```python
from build123d import *

# Parameters (mm, degrees)
SPLIT_2_DEPTH      = 10
SPLIT_2_DEPTH_BACK = 40.867646096
SPLSKE_W           = 5.7748
SPLSKE_H           = 1.850215418


with BuildPart() as part:
    # BodySke → Body (revolve)
    with BuildSketch(Plane.XY, mode=Mode.PRIVATE) as body_sk:
        with BuildLine():
            Line((0, 2.5), (38.74, 2.8874))
            ThreePointArc((38.74, 2.8874), (39.422958568, 1.514905806), (39.65797584, 0))
            Line((39.65797584, 0), (-0.669872981, 0))
            ThreePointArc((-0.669872981, 0), (-0.499502113, 1.294095226), (0, 2.5))
        make_face()
    revolve(body_sk.sketch.rotate(Axis((-0.669872981, 0, 0), (1, 0, 0)), 90), axis=Axis((-0.669872981, 0, 0), (1, 0, 0)))

    # SplSke → Split 2 (cut, two sides: drawn at the far end of the back side and taken through both)
    with BuildSketch(Plane(origin=(0, 0, 0), x_dir=(0, 0, -1), z_dir=(1, 0, 0)).offset(-SPLIT_2_DEPTH_BACK)):
        Rectangle(SPLSKE_W, SPLSKE_H)
    extrude(amount=SPLIT_2_DEPTH + SPLIT_2_DEPTH_BACK, mode=Mode.SUBTRACT)


solid = part.part
```
Verification items for the finished model (mm, model axes). Coordinates: 2 decimals unless noted, no trailing zeros. Loops run counter-clockwise (first coordinate to the right, second up) from the corner with the lowest first, then second, coordinate; pieces in that order, holes last. Notation, with made-up numbers: (44.5, 66.5) -> (65.5, 66.5) arc R21 ccw to (65.5, 100.5) -> close; hole circle Ø5 at (2.25, 73). An arc over 180 degrees is marked (long way). Put each result on its own line as item: value.
1. Gauge pin test, flat ends, axial feed: P1, Ø1.5, axis at x = 3.5, z = 0.5, coming from the -Y side; P2, Ø1, axis at x = 8.5, y = 2, coming from the -Z side; P3, Ø2, axis at y = 0.5, z = -1, coming from the +X side; P4, Ø2, axis at y = 0.5, z = 0.5, coming from the -X side. Record the tip position at first contact, or that the pin passes through.
Result set:
P1: stops at y = -2.54
P2: stops at z = -2.11
P3: stops at x = 39.66
P4: stops at x = -0.58
2. Mould release check, pull along Y, two halves, no side actions. Record for faces 1 (the face through (5, -0.925, 0)), 2 (the face through (19.641, 2.392, 1.244)): pulls with the +Y half, pulls with the -Y half, needs draft (parallel to the pull), parting line crosses it, or undercut.
Result set:
face 1: undercut
face 2: parting line crosses it
3. Section check B-B, the plane x = 34. Record the boundary of the cut face in (y, z).
Result set:
outline: circle Ø5.68 at (0, 0)
4. Section check A-A, the plane x = 5.5. Record the boundary of the cut face in (y, z) (3 decimals), then the cut area to 3 significant figures.
Result set:
outline: (-0.925, -2.382) -> (-0.925, 2.382) arc R2.555 ccw to start; (0.925, -2.382) arc R2.555 ccw to (0.925, 2.382) -> close
area: 11.3 mm^2
5. Section check C-C, the plane x = 18. Record the boundary of the cut face in (y, z).
Result set:
outline: circle Ø5.36 at (0, 0)
6. Thickness scan on line 1 (Y direction, x = 8, z = -0.6); line 2 (Y direction, x = 2, z = 1.75); line 3 (Y direction, x = 23, z = 1.3). Record the ranges inside material, lowest first.
Result set:
line 1: y = -2.51 to -0.93, 0.93 to 2.51
line 2: y = -1.81 to -0.93, 0.93 to 1.81
line 3: y = -2.4 to 2.4
